Can you work these out from the drawing? Everything is in mm from the part's minimum corner. Round coordinates to 2 decimals unless told otherwise and drop trailing zeros. Loops run counter-clockwise (first coordinate to the right, second up) from the corner with the lowest first, then second, coordinate; pieces in that order, holes last. Notation, with made-up numbers: (26, -17.5) - (43, -17.5) arc R19 cw to (43, -0.5) - close; hole circle Ø3 at (-7, -4). An arc over 180 degrees is marked (long way). Return JSON: item names as keys, results as strings. Group by question number.
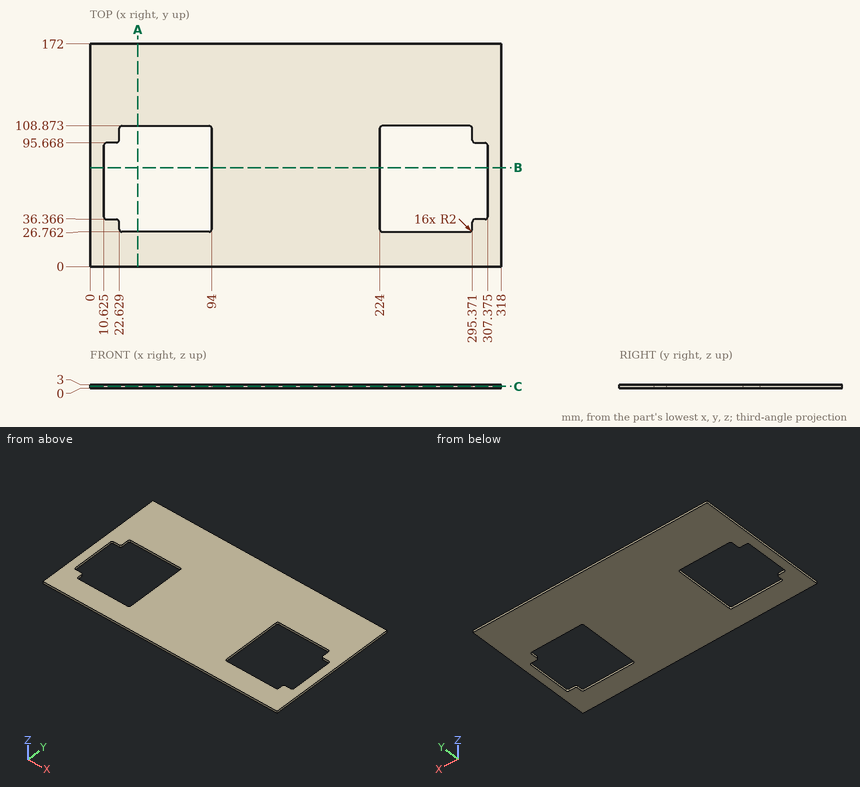
Q1. Will this pin go through, and if not, where does the flat tip stop? pin 1 Ø1.5 at (x, y) = (286, 29.5) entering from +Z.
Q2. Imagine slicing it at C-C, the plane z = 1.6. Give the number of separate pieces and of enclosed holes in the cut face, and give its area (3 significant figures).
Q3. Imagine slicing it at B-B, the plane y = 76.5. List the corners of the cut face in (x, z) for me (1 decimal).
Q4. Imagine slicing it at A-A, the plane x = 37. List the corners of the cut face in (y, z) for me.
Q5. Please list where these lines run through material, in increasing order: line 1 (X direction, y = 60, z = 1.9) (1 decimal); line 2 (Y direction, x = 302, z = 0.4); line 3 (Y direction, x = 287.5, z = 1.55).
Output values:
{
 "1": {"pin 1": "passes through"},
 "2": {"separate pieces": "1", "enclosed holes": "2", "area": "41,600 mm^2"},
 "3": {"outline": "(0, 0) - (10.6, 0) - (10.6, 3) - (0, 3) - close; (94, 0) - (224, 0) - (224, 3) - (94, 3) - close; (307.4, 0) - (318, 0) - (318, 3) - (307.4, 3) - close"},
 "4": {"outline": "(0, 0) - (26.76, 0) - (26.76, 3) - (0, 3) - close; (108.87, 0) - (172, 0) - (172, 3) - (108.87, 3) - close"},
 "5": {"line 1": "x = 0 to 10.6, 94 to 224, 307.4 to 318", "line 2": "y = 0 to 36.37, 95.67 to 172", "line 3": "y = 0 to 26.76, 108.87 to 172"}
}
